```python
from build123d import *

# Parameters (mm, degrees)
SKETCH1_W                                           = 60
SKETCH1_H                                           = 10
BOSS_EXTRUDE1_DEPTH                                 = 3
CSK_FOR_M3_COUNTERSUNK_FLAT_HEAD_SCREW1_D           = 3.4
CSK_FOR_M3_COUNTERSUNK_FLAT_HEAD_SCREW1_DEPTH       = 7.5
CSK_FOR_M3_COUNTERSUNK_FLAT_HEAD_SCREW1_CSINK_D     = 6.3
CSK_FOR_M3_COUNTERSUNK_FLAT_HEAD_SCREW1_CSINK_ANGLE = 90
CSK_FOR_M3_COUNTERSUNK_FLAT_HEAD_SCREW1_TIP         = 1.021463052
SKETCH4_W                                           = 5
SKETCH4_H                                           = 1.5
CUT_EXTRUDE1_DEPTH                                  = 8.5


with BuildPart() as part:
    # Sketch1 → Boss-Extrude1 (new body)
    with BuildSketch(Plane(origin=(0, 0, 0), x_dir=(1, 0, 0), z_dir=(0, 1, 0))):
        Rectangle(SKETCH1_W, SKETCH1_H)
    extrude(amount=BOSS_EXTRUDE1_DEPTH)

    # CSK for M3 Countersunk Flat Head Screw1
    with Locations(Plane(origin=(-15, 3, 0), x_dir=(0, 0, 1), z_dir=(0, 1, 0))):
        with Locations((0, 0), (0, 30)):
            CounterSinkHole(CSK_FOR_M3_COUNTERSUNK_FLAT_HEAD_SCREW1_D / 2, CSK_FOR_M3_COUNTERSUNK_FLAT_HEAD_SCREW1_CSINK_D / 2, depth=CSK_FOR_M3_COUNTERSUNK_FLAT_HEAD_SCREW1_DEPTH, counter_sink_angle=CSK_FOR_M3_COUNTERSUNK_FLAT_HEAD_SCREW1_CSINK_ANGLE)
            with Locations((0, 0, -(CSK_FOR_M3_COUNTERSUNK_FLAT_HEAD_SCREW1_DEPTH + CSK_FOR_M3_COUNTERSUNK_FLAT_HEAD_SCREW1_TIP / 2))):  # 118° drill point
                Cone(0, CSK_FOR_M3_COUNTERSUNK_FLAT_HEAD_SCREW1_D / 2, CSK_FOR_M3_COUNTERSUNK_FLAT_HEAD_SCREW1_TIP, mode=Mode.SUBTRACT)

    # Sketch4 → Cut-Extrude1 (cut)
    with BuildSketch(Plane.XY.offset(5)):
        with Locations((0, 0.75)):
            Rectangle(SKETCH4_W, SKETCH4_H)
    extrude(amount=-CUT_EXTRUDE1_DEPTH, mode=Mode.SUBTRACT)


solid = part.part
```
Build history of the part. All positions in model axes, mm. A direction names the side the tool comes from. Give positions to 0.01 mm unless a question says otherwise; leave off trailing zeros. Loops run counter-clockwise (first coordinate to the right, second up) from the corner with the lowest first, then second, coordinate; pieces in that order, holes last.
Item 1: Flat gauge pins, fed straight in: pin 1 (1.5 mm diameter, centred on x = -1, z = 1, fed in from -Y); pin 2 (1.6 mm diameter, centred on x = 0.5, y = 0.5, fed in from +Z). Where does each tip first touch, or does it go through?
Answers follow:
pin 1: stops at y = 1.5
pin 2: stops at z = -3.5
Item 2: Pull direction Z, two halves, no side cores. Call faces 1 (the face through (13.34, 0.76, 0.37)), 2 (the face through (-13.314, 0.764, 0.221)), 3 (the face through (0, 1, -3.5)), 4 (the face through (-30, 1, 0)): released by +Z, released by -Z, zero draft, split by the parting line, or undercut.
Answers follow:
face 1: undercut
face 2: undercut
face 3: released by +Z
face 4: zero draft
Item 3: Slice it at C-C, the plane z = 0. List the corners of the cut face in (x, y).
Answers follow:
outline: (-30, 0) - (-16.7, 0) - (-16.7, 1.55) - (-18.15, 3) - (-30, 3) - close; (-13.3, 0) - (-2.5, 0) - (-2.5, 1.5) - (2.5, 1.5) - (2.5, 0) - (13.3, 0) - (13.3, 1.55) - (11.85, 3) - (-11.85, 3) - (-13.3, 1.55) - close; (16.7, 0) - (30, 0) - (30, 3) - (18.15, 3) - (16.7, 1.55) - close
Item 4: Drill centre lines: line 1 (X direction, y = 0.65, z = 0); line 2 (X direction, y = 2.75, z = 1.75); line 3 (Z direction, x = -15, y = 0.55). Where is each one in solid material? Low to high.
Answers follow:
line 1: x = -30 to -16.7, -13.3 to -2.5, 2.5 to 13.3, 16.7 to 30
line 2: x = -30 to -17.31, -12.69 to 12.69, 17.31 to 30
line 3: z = -5 to -1.7, 1.7 to 5
Item 5: Slice it at A-A, the plane x = 15. List the corners of the cut face in (y, z), and give its area (3 significant figures).
Answers follow:
outline: (0, -5) - (3, -5) - (3, -3.15) - (1.55, -1.7) - (0, -1.7) - close; (0, 1.7) - (1.55, 1.7) - (3, 3.15) - (3, 5) - (0, 5) - close
area: 17.7 mm2
Item 6: Slice it at B-B, the plane y = 0.45. List the corners of the cut face in (x, z), and give its area (3 significant figures).
Answers follow:
outline: (-30, -5) - (30, -5) - (30, 5) - (2.5, 5) - (2.5, -3.5) - (-2.5, -3.5) - (-2.5, 5) - (-30, 5) - close; hole circle Ø3.4 at (-15, 0); hole circle Ø3.4 at (15, 0)
area: 539 mm2
Item 7: Which spindle directions (+Z, -Z, +X, -X, +Y, -Y) get a long thin tool onto all of the face, cutting with end or side? Do faces 5 (the face through (0, 1.5, 1)), 6 (the face through (-0.4, 0, -4.5)). Say none if no direction does.
Answers follow:
face 5: +Z, -Y
face 6: +Z, -Z, +X, -X, -Y
